from build123d import *

# Parameters (mm, degrees)
SKETCH2_W           = 60
SKETCH2_H           = 25
SKETCH2_R           = 3.3
BOSS_EXTRUDE2_DEPTH = 5
SKETCH3_W           = 5
SKETCH3_H           = 48
BOSS_EXTRUDE3_DEPTH = 25
CUT_EXTRUDE1_REACH  = 72.801
SKETCH5_W           = 14.75
SKETCH5_H           = 25
BOSS_EXTRUDE4_DEPTH = 5
CHAMFER1_SIZE       = 2
CHAMFER2_SIZE       = 5
CHAMFER3_SIZE       = 1


with BuildPart() as part:
    # Sketch2 → Boss-Extrude2 (new body)
    with BuildSketch(Plane(origin=(0, 0, 0), x_dir=(1, 0, 0), z_dir=(0, 1, 0))):
        Rectangle(SKETCH2_W, SKETCH2_H)
        with Locations(Location((-23, 6.5, 0), (0, 0, 270))):
            Circle(SKETCH2_R, mode=Mode.SUBTRACT)
        with Locations(Location((23, 6.5, 0), (0, 0, 270))):
            Circle(SKETCH2_R, mode=Mode.SUBTRACT)
        with Locations(Location((-23, -6.5, 0), (0, 0, 270))):
            Circle(SKETCH2_R, mode=Mode.SUBTRACT)
        with Locations(Location((23, -6.5, 0), (0, 0, 270))):
            Circle(SKETCH2_R, mode=Mode.SUBTRACT)
    extrude(amount=BOSS_EXTRUDE2_DEPTH)

    # Sketch3 → Boss-Extrude3 (add)
    with BuildSketch(Plane.XY.offset(12.5)):
        with Locations((-12.75, 29)):
            Rectangle(SKETCH3_W, SKETCH3_H)
        with Locations((12.75, 29)):
            Rectangle(SKETCH3_W, SKETCH3_H)
    extrude(amount=-BOSS_EXTRUDE3_DEPTH)

    # Cut-Extrude1: up to this face of the body (flat: up to its plane)
    cut_extrude1_end = Plane(part.part.faces().sort_by_distance((-15.25, 29, 0))[0])
    # Sketch4 → Cut-Extrude1 (cut, up to the picked face)
    with BuildSketch(Plane(origin=(15.25, 0, 0), x_dir=(0, 0, -1), z_dir=(1, 0, 0)), mode=Mode.PRIVATE) as cut_extrude1_sk1:
        with BuildLine():
            Line((2.6, 45.5), (2.6, 40.5))
            ThreePointArc((2.6, 40.5), (0, 37.9), (-2.6, 40.5))
            Line((-2.6, 40.5), (-2.6, 45.5))
            ThreePointArc((-2.6, 45.5), (0, 48.1), (2.6, 45.5))
        make_face()
    cut_extrude1_tool1 = split(extrude(cut_extrude1_sk1.sketch, amount=-CUT_EXTRUDE1_REACH, mode=Mode.PRIVATE), bisect_by=cut_extrude1_end, keep=Keep.BOTH, mode=Mode.PRIVATE)
    add(cut_extrude1_tool1.solids().sort_by(Axis((15.25, 43, 0), (-1, 0, 0)))[0], mode=Mode.SUBTRACT)

    # Sketch5 → Boss-Extrude4 (add)
    # profile 1 of 2: a face of its own
    with BuildSketch(Plane(origin=(0, 5, 0), x_dir=(1, 0, 0), z_dir=(0, 1, 0))):
        with Locations((22.625, 0)):
            Rectangle(SKETCH5_W, SKETCH5_H)
        Polygon((28.773502692, 6.5), (25.886751346, 11.5), (20.113248654, 11.5), (17.226497308, 6.5), (20.113248654, 1.5), (25.886751346, 1.5), align=None, mode=Mode.SUBTRACT)
        Polygon((25.886751346, -1.5), (28.773502692, -6.5), (25.886751346, -11.5), (20.113248654, -11.5), (17.226497308, -6.5), (20.113248654, -1.5), align=None, mode=Mode.SUBTRACT)
    # profile 2 of 2: a face of its own
    with BuildSketch(Plane(origin=(0, 5, 0), x_dir=(1, 0, 0), z_dir=(0, 1, 0))):
        with Locations((-22.625, 0)):
            Rectangle(SKETCH5_W, SKETCH5_H)
        Polygon((-17.226497308, 6.5), (-20.113248654, 11.5), (-25.886751346, 11.5), (-28.773502692, 6.5), (-25.886751346, 1.5), (-20.113248654, 1.5), align=None, mode=Mode.SUBTRACT)
        Polygon((-20.113248654, -1.5), (-17.226497308, -6.5), (-20.113248654, -11.5), (-25.886751346, -11.5), (-28.773502692, -6.5), (-25.886751346, -1.5), align=None, mode=Mode.SUBTRACT)
    extrude(amount=BOSS_EXTRUDE4_DEPTH)

    # Chamfer1
    # the kernel refuses this chamfer: 2 mm, written as the material it adds along each edge
    with BuildSketch(Plane(origin=(15.25, 10, -12.5), x_dir=(0.9996219169112968, -0.02749587661058651, 0), z_dir=(0, 0, 1))) as chamfer1_piece_1_section:
        Polygon((CHAMFER1_SIZE * 0.999621916911, CHAMFER1_SIZE * 0.0274958766106), (-CHAMFER1_SIZE * 0.0274958766106, CHAMFER1_SIZE * 0.999621916911), (0, 0), align=None)
    chamfer1_piece_1 = extrude(amount=25, mode=Mode.PRIVATE)
    chamfer1_piece_1 = split(chamfer1_piece_1, bisect_by=Plane(origin=(15.178146825, 10.596401608, -10.047847108), z_dir=(0.8660254037844565, 0, -0.4999999999999692)), keep=Keep.TOP, mode=Mode.PRIVATE)
    chamfer1_piece_1 = split(chamfer1_piece_1, bisect_by=Plane(origin=(18.675487588, 10.596401608, -9.009724784), z_dir=(-0.8660254037844565, 0, -0.49999999999996914)), keep=Keep.TOP, mode=Mode.PRIVATE)
    add(chamfer1_piece_1)
    with BuildSketch(Plane(origin=(15.25, 10, -12.5), x_dir=(0.9996219169112968, -0.02749587661058651, 0), z_dir=(0, 0, 1))) as chamfer1_piece_2_section:
        Polygon((CHAMFER1_SIZE * 0.999621916911, CHAMFER1_SIZE * 0.0274958766106), (-CHAMFER1_SIZE * 0.0274958766106, CHAMFER1_SIZE * 0.999621916911), (0, 0), align=None)
    chamfer1_piece_2 = extrude(amount=25, mode=Mode.PRIVATE)
    chamfer1_piece_2 = split(chamfer1_piece_2, bisect_by=Plane(origin=(16.849076721, 10.762644927, -7.153711633), z_dir=(-0.8660254037844565, 0, 0.4999999999999692)), keep=Keep.TOP, mode=Mode.PRIVATE)
    chamfer1_piece_2 = split(chamfer1_piece_2, bisect_by=Plane(origin=(16.849076721, 10.762644927, -5.846288367), z_dir=(-0.8660254037844565, 0, -0.49999999999996914)), keep=Keep.TOP, mode=Mode.PRIVATE)
    add(chamfer1_piece_2)
    with BuildSketch(Plane(origin=(15.25, 10, -12.5), x_dir=(0.9996219169112968, -0.02749587661058651, 0), z_dir=(0, 0, 1))) as chamfer1_piece_3_section:
        Polygon((CHAMFER1_SIZE * 0.999621916911, CHAMFER1_SIZE * 0.0274958766106), (-CHAMFER1_SIZE * 0.0274958766106, CHAMFER1_SIZE * 0.999621916911), (0, 0), align=None)
    chamfer1_piece_3 = extrude(amount=25, mode=Mode.PRIVATE)
    chamfer1_piece_3 = split(chamfer1_piece_3, bisect_by=Plane(origin=(14.108732703, 10.603890332, 1.099873298), z_dir=(0.8660254037844565, 0, -0.49999999999996914)), keep=Keep.TOP, mode=Mode.PRIVATE)
    chamfer1_piece_3 = split(chamfer1_piece_3, bisect_by=Plane(origin=(19.737897828, 10.603890332, 2.150126702), z_dir=(-0.8660254037844565, 0, -0.4999999999999692)), keep=Keep.TOP, mode=Mode.PRIVATE)
    chamfer1_piece_3 = split(chamfer1_piece_3, bisect_by=Plane(origin=(19.737897828, 10.603890332, -2.150126702), z_dir=(-0.8660254037844565, 0, 0.4999999999999692)), keep=Keep.TOP, mode=Mode.PRIVATE)
    chamfer1_piece_3 = split(chamfer1_piece_3, bisect_by=Plane(origin=(14.108732703, 10.603890332, -1.099873298), z_dir=(0.8660254037844565, 0, 0.49999999999996914)), keep=Keep.TOP, mode=Mode.PRIVATE)
    add(chamfer1_piece_3)
    with BuildSketch(Plane(origin=(15.25, 10, -12.5), x_dir=(0.9996219169112968, -0.02749587661058651, 0), z_dir=(0, 0, 1))) as chamfer1_piece_4_section:
        Polygon((CHAMFER1_SIZE * 0.999621916911, CHAMFER1_SIZE * 0.0274958766106), (-CHAMFER1_SIZE * 0.0274958766106, CHAMFER1_SIZE * 0.999621916911), (0, 0), align=None)
    chamfer1_piece_4 = extrude(amount=25, mode=Mode.PRIVATE)
    chamfer1_piece_4 = split(chamfer1_piece_4, bisect_by=Plane(origin=(16.849076721, 10.762644927, 5.846288367), z_dir=(-0.8660254037844565, 0, 0.49999999999996914)), keep=Keep.TOP, mode=Mode.PRIVATE)
    chamfer1_piece_4 = split(chamfer1_piece_4, bisect_by=Plane(origin=(16.849076721, 10.762644927, 7.153711633), z_dir=(-0.8660254037844565, 0, -0.4999999999999692)), keep=Keep.TOP, mode=Mode.PRIVATE)
    add(chamfer1_piece_4)
    with BuildSketch(Plane(origin=(15.25, 10, -12.5), x_dir=(0.9996219169112968, -0.02749587661058651, 0), z_dir=(0, 0, 1))) as chamfer1_piece_5_section:
        Polygon((CHAMFER1_SIZE * 0.999621916911, CHAMFER1_SIZE * 0.0274958766106), (-CHAMFER1_SIZE * 0.0274958766106, CHAMFER1_SIZE * 0.999621916911), (0, 0), align=None)
    chamfer1_piece_5 = extrude(amount=25, mode=Mode.PRIVATE)
    chamfer1_piece_5 = split(chamfer1_piece_5, bisect_by=Plane(origin=(18.675487588, 10.596401608, 9.009724784), z_dir=(-0.8660254037844565, 0, 0.49999999999996914)), keep=Keep.TOP, mode=Mode.PRIVATE)
    chamfer1_piece_5 = split(chamfer1_piece_5, bisect_by=Plane(origin=(15.178146825, 10.596401608, 10.047847108), z_dir=(0.8660254037844565, 0, 0.4999999999999692)), keep=Keep.TOP, mode=Mode.PRIVATE)
    add(chamfer1_piece_5)
    with BuildSketch(Plane(origin=(-15.25, 10, 12.5), x_dir=(0.027495876610586487, 0.9996219169112968, 0), z_dir=(0, 0, -1))) as chamfer1_piece_6_section:
        Polygon((CHAMFER1_SIZE * 0.999621916911, -CHAMFER1_SIZE * 0.0274958766106), (-CHAMFER1_SIZE * 0.0274958766106, -CHAMFER1_SIZE * 0.999621916911), (0, 0), align=None)
    chamfer1_piece_6 = extrude(amount=25, mode=Mode.PRIVATE)
    chamfer1_piece_6 = split(chamfer1_piece_6, bisect_by=Plane(origin=(-15.178146825, 10.596401608, 10.047847108), z_dir=(-0.866025403784439, 0, 0.4999999999999995)), keep=Keep.TOP, mode=Mode.PRIVATE)
    chamfer1_piece_6 = split(chamfer1_piece_6, bisect_by=Plane(origin=(-18.675487588, 10.596401608, 9.009724784), z_dir=(0.8660254037844384, 0, 0.5000000000000004)), keep=Keep.TOP, mode=Mode.PRIVATE)
    add(chamfer1_piece_6)
    with BuildSketch(Plane(origin=(-15.25, 10, 12.5), x_dir=(0.027495876610586487, 0.9996219169112968, 0), z_dir=(0, 0, -1))) as chamfer1_piece_7_section:
        Polygon((CHAMFER1_SIZE * 0.999621916911, -CHAMFER1_SIZE * 0.0274958766106), (-CHAMFER1_SIZE * 0.0274958766106, -CHAMFER1_SIZE * 0.999621916911), (0, 0), align=None)
    chamfer1_piece_7 = extrude(amount=25, mode=Mode.PRIVATE)
    chamfer1_piece_7 = split(chamfer1_piece_7, bisect_by=Plane(origin=(-16.849076721, 10.762644927, 7.153711633), z_dir=(0.866025403784439, 0, -0.4999999999999995)), keep=Keep.TOP, mode=Mode.PRIVATE)
    chamfer1_piece_7 = split(chamfer1_piece_7, bisect_by=Plane(origin=(-16.849076721, 10.762644927, 5.846288367), z_dir=(0.8660254037844384, 0, 0.5000000000000004)), keep=Keep.TOP, mode=Mode.PRIVATE)
    add(chamfer1_piece_7)
    with BuildSketch(Plane(origin=(-15.25, 10, 12.5), x_dir=(0.027495876610586487, 0.9996219169112968, 0), z_dir=(0, 0, -1))) as chamfer1_piece_8_section:
        Polygon((CHAMFER1_SIZE * 0.999621916911, -CHAMFER1_SIZE * 0.0274958766106), (-CHAMFER1_SIZE * 0.0274958766106, -CHAMFER1_SIZE * 0.999621916911), (0, 0), align=None)
    chamfer1_piece_8 = extrude(amount=25, mode=Mode.PRIVATE)
    chamfer1_piece_8 = split(chamfer1_piece_8, bisect_by=Plane(origin=(-19.737897828, 10.603890332, 2.150126702), z_dir=(0.866025403784439, 0, -0.4999999999999995)), keep=Keep.TOP, mode=Mode.PRIVATE)
    chamfer1_piece_8 = split(chamfer1_piece_8, bisect_by=Plane(origin=(-14.108732703, 10.603890332, 1.099873298), z_dir=(-0.8660254037844384, 0, -0.5000000000000004)), keep=Keep.TOP, mode=Mode.PRIVATE)
    chamfer1_piece_8 = split(chamfer1_piece_8, bisect_by=Plane(origin=(-14.108732703, 10.603890332, -1.099873298), z_dir=(-0.8660254037844384, 0, 0.5000000000000006)), keep=Keep.TOP, mode=Mode.PRIVATE)
    chamfer1_piece_8 = split(chamfer1_piece_8, bisect_by=Plane(origin=(-19.737897828, 10.603890332, -2.150126702), z_dir=(0.866025403784439, 0, 0.4999999999999995)), keep=Keep.TOP, mode=Mode.PRIVATE)
    add(chamfer1_piece_8)
    with BuildSketch(Plane(origin=(-15.25, 10, 12.5), x_dir=(0.027495876610586487, 0.9996219169112968, 0), z_dir=(0, 0, -1))) as chamfer1_piece_9_section:
        Polygon((CHAMFER1_SIZE * 0.999621916911, -CHAMFER1_SIZE * 0.0274958766106), (-CHAMFER1_SIZE * 0.0274958766106, -CHAMFER1_SIZE * 0.999621916911), (0, 0), align=None)
    chamfer1_piece_9 = extrude(amount=25, mode=Mode.PRIVATE)
    chamfer1_piece_9 = split(chamfer1_piece_9, bisect_by=Plane(origin=(-16.849076721, 10.762644927, -5.846288367), z_dir=(0.8660254037844384, 0, -0.5000000000000006)), keep=Keep.TOP, mode=Mode.PRIVATE)
    chamfer1_piece_9 = split(chamfer1_piece_9, bisect_by=Plane(origin=(-16.849076721, 10.762644927, -7.153711633), z_dir=(0.866025403784439, 0, 0.4999999999999995)), keep=Keep.TOP, mode=Mode.PRIVATE)
    add(chamfer1_piece_9)
    with BuildSketch(Plane(origin=(-15.25, 10, 12.5), x_dir=(0.027495876610586487, 0.9996219169112968, 0), z_dir=(0, 0, -1))) as chamfer1_piece_10_section:
        Polygon((CHAMFER1_SIZE * 0.999621916911, -CHAMFER1_SIZE * 0.0274958766106), (-CHAMFER1_SIZE * 0.0274958766106, -CHAMFER1_SIZE * 0.999621916911), (0, 0), align=None)
    chamfer1_piece_10 = extrude(amount=25, mode=Mode.PRIVATE)
    chamfer1_piece_10 = split(chamfer1_piece_10, bisect_by=Plane(origin=(-18.675487588, 10.596401608, -9.009724784), z_dir=(0.8660254037844384, 0, -0.5000000000000006)), keep=Keep.TOP, mode=Mode.PRIVATE)
    chamfer1_piece_10 = split(chamfer1_piece_10, bisect_by=Plane(origin=(-15.178146825, 10.596401608, -10.047847108), z_dir=(-0.866025403784439, 0, -0.4999999999999995)), keep=Keep.TOP, mode=Mode.PRIVATE)
    add(chamfer1_piece_10)

    # Chamfer2
    chamfer2_edges = [part.edges().sort_by_distance(p)[0] for p in [
        (-10.25, 5, 0),
        (10.25, 5, 0),
    ]]
    chamfer(chamfer2_edges, length=CHAMFER2_SIZE)

    # Chamfer3
    chamfer3_edges = [part.edges().sort_by_distance(p)[0] for p in [
        (30, 5, 12.5),
        (-30, 5, 12.5),
        (-30, 5, -12.5),
        (30, 5, -12.5),
    ]]
    chamfer(chamfer3_edges, length=CHAMFER3_SIZE)


solid = part.part
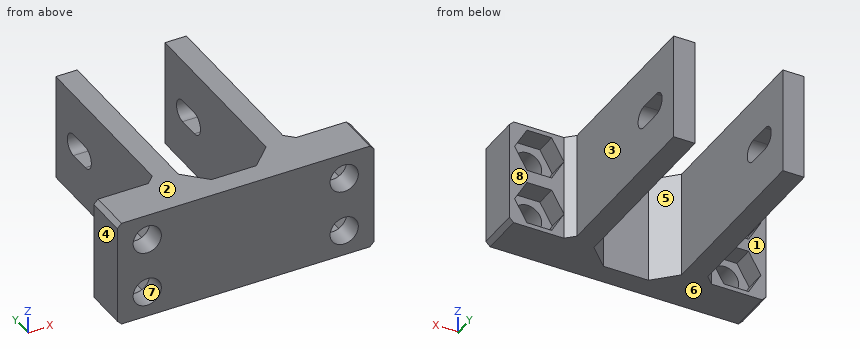
Geometry: final body of the model. Coordinates: model frame, mm. Face numbers are marked on the shaded views. A direction names the side the tool comes from. Coordinates: 2 decimals unless noted, no trailing zeros. Loops run counter-clockwise (first coordinate to the right, second up) from the corner with the lowest first, then second, coordinate; pieces in that order, holes last. Notation, with made-up numbers: (12.5, 15.5) - (68.5, 15.5) arc R22 ccw to (68.5, 22.5) - close; hole circle Ø11 at (-15, 34). An arc over 180 degrees is marked (long way). One line per question, with ' | ' between items. Start each with the question number.
(1) Reachability of the marked faces 1, 2, 3, 4 and 5 from +Z, -Z, +X, -X, +Y, -Y: full face, straight path, thin tool, end or side. Return the list, or none.
(2) Cut plane A-A on y = 42. Output: boundary loops of the cut face in (x, z).
(3) Ray query, L1, parallel to X at y = 2.3, z = -6.5; L2, parallel to X at y = 32.5, z = -4; L3, parallel to Z at x = -20.5, y = 6.5. Return the intervals inside material, ascending. Write a range as from..to.
(4) Draft query along Z for the marked faces 6, 7 and 8. Return one class per face: +Z half, -Z half, draft (parallel to the pull), parting line (faces both ways), or undercut.
(5) Cut plane C-C on z = 0. Output: boundary loops of the cut face in (x, y).
(6) Cut plane B-B on x = 23. Output: boundary loops of the cut face in (y, z).
(7) First-contact query: pin 1 (10 mm diameter, centred on x = 20.5, y = 32.5, fed in from -Z); pin 2 (7.5 mm diameter, centred on y = 38, z = 4.5, fed in from -X); pin 3 (6 mm diameter, centred on y = 46, z = 4, fed in from -X); pin 4 (8 mm diameter, centred on x = 22.5, z = -7, fed in from +Y). Flat tips, straight axial feed; report the tip coordinate or a pass-through.
(8) Cut plane D-D on y = 14. Output: boundary loops of the cut face in (x, z), and give its area (3 significant figures).
Here are the results:
1) face 1: +Z, -Z, -X, +Y | face 2: +Z, +X, -X, +Y, -Y | face 3: +Z, -Z, +X, +Y | face 4: +Z, -Z, -X, +Y, -Y | face 5: +Z, -Z, +Y
2) outline: (-15.25, -12.5) - (-10.25, -12.5) - (-10.25, -2.6) - (-15.25, -2.6) - close; (-15.25, 2.6) - (-10.25, 2.6) - (-10.25, 12.5) - (-15.25, 12.5) - close; (10.25, -12.5) - (15.25, -12.5) - (15.25, -2.6) - (10.25, -2.6) - close; (10.25, 2.6) - (15.25, 2.6) - (15.25, 12.5) - (10.25, 12.5) - close
3) L1: -30..-26.3, -19.7..19.7, 26.3..30 | L2: -15.25..-10.25, 10.25..15.25 | L3: -12.5..-11.5, -1.5..1.5, 11.5..12.5
4) face 6: -Z half | face 7: undercut | face 8: draft
5) outline: (-30, 0) - (30, 0) - (30, 10) - (17.25, 10) - (15.25, 12) - (15.25, 37.9) - (10.25, 37.9) - (10.25, 10) - (5.25, 5) - (-5.25, 5) - (-10.25, 10) - (-10.25, 37.9) - (-15.25, 37.9) - (-15.25, 12) - (-17.25, 10) - (-30, 10) - close; (-15.25, 48.1) - (-10.25, 48.1) - (-10.25, 53) - (-15.25, 53) - close; (10.25, 48.1) - (15.25, 48.1) - (15.25, 53) - (10.25, 53) - close
6) outline: (0, -12.5) - (10, -12.5) - (10, -11.5) - (5, -11.5) - (5, -9.8) - (0, -9.8) - close; (0, -3.2) - (5, -3.2) - (5, -1.5) - (10, -1.5) - (10, 1.5) - (5, 1.5) - (5, 3.2) - (0, 3.2) - close; (0, 9.8) - (5, 9.8) - (5, 11.5) - (10, 11.5) - (10, 12.5) - (0, 12.5) - close
7) pin 1: through | pin 2: x = -15.25 | pin 3: x = -15.25 | pin 4: y = 5
8) outline: (-15.25, -12.5) - (-10.25, -12.5) - (-10.25, 12.5) - (-15.25, 12.5) - close; (10.25, -12.5) - (15.25, -12.5) - (15.25, 12.5) - (10.25, 12.5) - close | area: 250 mm²
